Source: CAD feature listing. Evaluate the final solid. Frame: model axes, mm. Face numbers are marked on the shaded views. A direction names the side the tool comes from. Coordinates: 2 decimals unless noted, no trailing zeros. Loops run counter-clockwise (first coordinate to the right, second up) from the corner with the lowest first, then second, coordinate; pieces in that order, holes last. Notation, with made-up numbers: (36.5, 88.5) -> (94.5, 88.5) arc R10 ccw to (94.5, 107.5) -> close; hole circle Ø5 at (58.25, -39). An arc over 180 degrees is marked (long way). Answer as a JSON object with one key per item and string values. Group by question number.
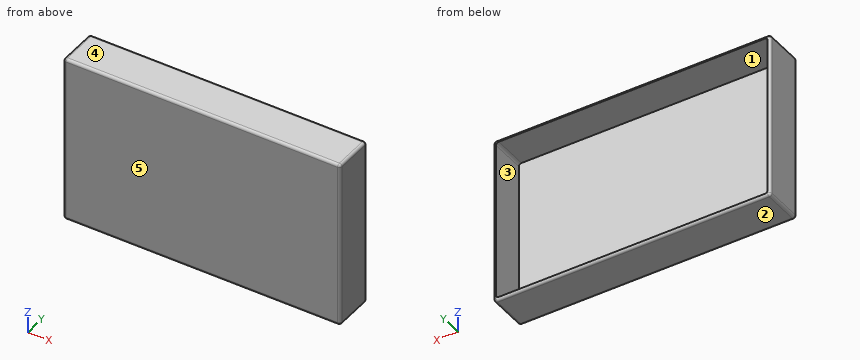
from build123d import *

# Parameters (mm, degrees)
SKETCH1_W           = 102
SKETCH1_H           = 62
BOSS_EXTRUDE1_DEPTH = 15
SKETCH2_W           = 100
SKETCH2_H           = 60
CUT_EXTRUDE1_DEPTH  = 13
FILLET2_R           = 1
FILLET3_R           = 1


with BuildPart() as part:
    # Sketch1 → Boss-Extrude1 (new body)
    with BuildSketch(Plane(origin=(0, 0, 0), x_dir=(1, 0, 0), z_dir=(0, 1, 0))):
        Rectangle(SKETCH1_W, SKETCH1_H)
    extrude(amount=BOSS_EXTRUDE1_DEPTH)

    # Sketch2 → Cut-Extrude1 (cut)
    with BuildSketch(Plane(origin=(0, 15, 0), x_dir=(1, 0, 0), z_dir=(0, 1, 0))):
        Rectangle(SKETCH2_W, SKETCH2_H)
    extrude(amount=-CUT_EXTRUDE1_DEPTH, mode=Mode.SUBTRACT)

    # Fillet2
    fillet2_edges = [part.edges().sort_by_distance(p)[0] for p in [
        (50, 8.5, -30),
        (50, 8.5, 30),
        (-50, 8.5, 30),
        (-50, 8.5, -30),
    ]]
    fillet(fillet2_edges, radius=FILLET2_R)

    # Fillet3
    fillet3_edges = [part.edges().sort_by_distance(p)[0] for p in [
        (-51, 15, 0),
        (0, 15, 31),
        (51, 15, 0),
        (0, 0, 31),
        (-51, 0, 0),
        (0, 0, -31),
        (51, 0, 0),
        (51, 7.5, 31),
        (-51, 7.5, 31),
        (-51, 7.5, -31),
        (51, 7.5, -31),
        (0, 15, -31),
    ]]
    fillet(fillet3_edges, radius=FILLET3_R - 0.0001)  # a hair under: the kernel refuses the full size


solid = part.part
1. Reachability of the marked faces 1 and 2 from +Z, -Z, +X, -X, +Y, -Y: full face, straight path, thin tool, end or side. Return the list, or none.
2. Section query A-A on y = 6.25. Return loops of the section in (x, z), then the cut area to 3 significant figures.
3. Pin query (flat end, axial travel): pin 1 Ø6 at (x, z) = (-6, 16) entering from +Y. Return the tip coordinate at first contact, or that it passes through.
4. Mould query, pull axis Z, two halves, no side actions, for the marked faces 3, 4 and 5. Classes: pulls with the +Z half, pulls with the -Z half, needs draft (parallel to the pull), parting line crosses it, or undercut.
5. Ray query, L1, parallel to X at y = 13.75, z = 6; L2, parallel to Z at x = -6, y = 8.75; L3, parallel to Y at x = -6, z = 25. Return the intervals inside material, ascending.
Solved:
{
 "1": {"face 1": "+Y", "face 2": "-Z, +X, -X, +Y, -Y"},
 "2": {"outline": "(-51, -30) arc R1 ccw to (-50, -31) -> (50, -31) arc R1 ccw to (51, -30) -> (51, 30) arc R1 ccw to (50, 31) -> (-50, 31) arc R1 ccw to (-51, 30) -> close; hole (-50, -29) arc R1 ccw to (-49, -30) -> (49, -30) arc R1 ccw to (50, -29) -> (50, 29) arc R1 ccw to (49, 30) -> (-49, 30) arc R1 ccw to (-50, 29) -> close", "area": "324 mm^2"},
 "3": {"pin 1": "y = 2"},
 "4": {"face 3": "undercut", "face 4": "pulls with the +Z half", "face 5": "needs draft"},
 "5": {"L1": "-51 to -50, 50 to 51", "L2": "-31 to -30, 30 to 31", "L3": "0 to 2"}
}
